Part model, mm, in its own coordinate system. Coordinates: 2 decimals unless noted, no trailing zeros. Write each loop counter-clockwise with the first axis right and the second up, starting at its lowest first coordinate (ties: lowest second). Pieces come first, ordered by that corner, then holes. Notation, with made-up numbers: (72, -28) - (118, -28) arc R34 cw to (118, 2) - close; hole circle Ø11 at (88.25, 84). An arc over 180 degrees is marked (long way). Use a Markdown table: item, result.
```python
from build123d import *

# Parameters (mm, degrees)
F0_W     = 89.054606
F0_H     = 77.087894
F1_DEPTH = 45.2606
F3_DEPTH = 90.5222
F4_R     = 16.270779
F5_DEPTH = 46.09548


with BuildPart() as f1:
    # F0 (on Front) → F1 (new body, symmetric)
    with BuildSketch(Plane.XZ):
        Rectangle(F0_W, F0_H)
    extrude(amount=F1_DEPTH, both=True)

    # F2 (on face) → F3 (cut, through all)
    with BuildSketch(Plane.XZ.offset(45.2606)):
        Polygon((44.527303, 38.543947), (0, 38.543947), (44.527303, 0), align=None)
    extrude(amount=-F3_DEPTH, mode=Mode.SUBTRACT)

    # F4 (on Front) → F5 (cut, symmetric)
    with BuildSketch(Plane.XZ):
        Circle(F4_R)
    extrude(amount=F5_DEPTH, both=True, mode=Mode.SUBTRACT)


solid = f1.part
```
Item 1: Band-saw the part on B-B, the plane y = 21. Give the cut face in (x, z).
From the geometry:
| item | result |
|---|---|
| outline | (-44.53, -38.54) - (44.53, -38.54) - (44.53, 0) - (0, 38.54) - (-44.53, 38.54) - close; hole circle Ø32.54 at (0, 0) |
Item 2: Band-saw the part on A-A, the plane x = 13. Give the cut face in (y, z).
From the geometry:
| item | result |
|---|---|
| outline | (-45.26, -38.54) - (45.26, -38.54) - (45.26, -9.78) - (-45.26, -9.78) - close; (-45.26, 9.78) - (45.26, 9.78) - (45.26, 27.29) - (-45.26, 27.29) - close |
Item 3: Band-saw the part on D-D, the plane z = 29. Give the cut face in (x, y).
From the geometry:
| item | result |
|---|---|
| outline | (-44.53, -45.26) - (11.03, -45.26) - (11.03, 45.26) - (-44.53, 45.26) - close |
Item 4: Two-plate mould, pull along X, no slides. Class faces 1 (the face through (22, -0.6, 19.5)), 2 (the face through (-23, -1, 38.544)), 3 (the face through (15.52, -0.63, 4.89)), 4 (the face through (-44.527, -1, -1)): pulls with the +X half, pulls with the -X half, needs draft (parallel to the pull), parting line crosses it, or undercut.
From the geometry:
| item | result |
|---|---|
| face 1 | pulls with the +X half |
| face 2 | needs draft |
| face 3 | undercut |
| face 4 | pulls with the -X half |
Item 5: Drop flat-ended pins along their axis: P1, Ø10, axis at x = 22, y = -18, coming from the +Z side; P2, Ø4, axis at y = -14.5, z = 10.5, coming from the +X side; P3, Ø6, axis at y = -6.5, z = 14.5, coming from the +X side. Give the stop position or say it passes through.
From the geometry:
| item | result |
|---|---|
| P1 | z = 23.83 |
| P2 | x = 34.71 |
| P3 | x = 31.24 |
Item 6: Drill centre lines: probe 1 along Z at (x, y) = (0, -7); probe 2 along Z at (x, y) = (-5, 10.5); probe 3 along X at (y, z) = (-41, 2). Where is each one in solid material? Low to high.
From the geometry:
| item | result |
|---|---|
| probe 1 | -38.54 to -16.27, 16.27 to 38.54 |
| probe 2 | -38.54 to -15.48, 15.48 to 38.54 |
| probe 3 | -44.53 to -16.15, 16.15 to 42.22 |
Item 7: Band-saw the part on C-C, the plane x = -15. Give the cut face in (y, z), then the cut area to 3 significant figures.
From the geometry:
| item | result |
|---|---|
| outline | (-45.26, -38.54) - (45.26, -38.54) - (45.26, -6.3) - (-45.26, -6.3) - close; (-45.26, 6.3) - (45.26, 6.3) - (45.26, 38.54) - (-45.26, 38.54) - close |
| area | 5,840 mm^2 |
